from build123d import *

# Parameters (mm, degrees)
SKETCH1_W           = 48
SKETCH1_H           = 59
BOSS_EXTRUDE1_DEPTH = 2
BOSS_EXTRUDE2_DEPTH = 59
SKETCH3_W           = 14
SKETCH3_H           = 55.8
CUT_EXTRUDE1_DEPTH  = 13


with BuildPart() as part:
    # Sketch1 → Boss-Extrude1 (new body)
    with BuildSketch(Plane.XY):
        Rectangle(SKETCH1_W, SKETCH1_H)
    extrude(amount=BOSS_EXTRUDE1_DEPTH)

    # Sketch2 → Boss-Extrude2 (add)
    with BuildSketch(Plane.XZ.offset(29.5)):
        with BuildLine():
            Line((-16, 15), (16, 15))
            ThreePointArc((16, 15), (21.656854249, 12.656854249), (24, 7))
            Line((24, 7), (24, 2))
            Line((24, 2), (-24, 2))
            Line((-24, 2), (-24, 7))
            ThreePointArc((-24, 7), (-21.656854249, 12.656854249), (-16, 15))
        make_face()
    extrude(amount=-BOSS_EXTRUDE2_DEPTH)

    # Sketch3 → Cut-Extrude1 (cut)
    with BuildSketch(Plane.XY.offset(15)):
        Rectangle(SKETCH3_W, SKETCH3_H)
        with Locations((15.4, 0)):
            Rectangle(SKETCH3_W, SKETCH3_H)
        with Locations((-15.4, 0)):
            Rectangle(SKETCH3_W, SKETCH3_H)
    extrude(amount=-CUT_EXTRUDE1_DEPTH, mode=Mode.SUBTRACT)


solid = part.part
Verification items for the finished model (mm, model axes). A direction names the side the tool comes from. Round coordinates to 2 decimals unless told otherwise and drop trailing zeros. Loops run counter-clockwise (first coordinate to the right, second up) from the corner with the lowest first, then second, coordinate; pieces in that order, holes last. Notation, with made-up numbers: M -21.5,36 L 4.5,36 A20 cw 4.5,52 Z; hole C 53.25,8 d4. An arc over 180 degrees is marked long. Write each question's results on one line, items separated by ' | '.
1) Section check A-A on z = 3. Record the boundary of the cut face in (x, y), then the cut area to 3 significant figures.
Checks:
outline: M -24,-29.5 L 24,-29.5 L 24,29.5 L -24,29.5 Z; hole M -22.4,-27.9 L -8.4,-27.9 L -8.4,27.9 L -22.4,27.9 Z; hole M -7,-27.9 L 7,-27.9 L 7,27.9 L -7,27.9 Z; hole M 8.4,-27.9 L 22.4,-27.9 L 22.4,27.9 L 8.4,27.9 Z | area: 488 mm2
2) Mould release check, pull along Y, two halves, no side actions. Record for faces 3 (the flat face through (-24, 0, 3)), 4 (the flat face through (0, 29.5, 8)), 5 (the flat face through (15, 27.9, 9)): released by +Y, released by -Y, zero draft, split by the parting line, or undercut.
Checks:
face 3: zero draft | face 4: released by +Y | face 5: undercut
3) Access from +Z, -Z, +X, -X, +Y, -Y to the whole of each face (thin tool, end or side, straight path). Record for faces 1 (the flat face through (7, 0, 9)), 2 (the cylindrical face through (23.213, -0.413, 10.46)).
Checks:
face 1: +Z | face 2: +Z, +X, +Y, -Y
4) Gauge pin test, flat ends, axial feed: P1, Ø1, axis at x = 3.5, y = -8.5, coming from the -Z side; P2, Ø11, axis at x = 16.5, y = 2, coming from the +Z side. Record the tip position at first contact, or that the pin passes through.
Checks:
P1: stops at z = 0 | P2: stops at z = 2
5) Section check D-D on z = 12.75. Record the boundary of the cut face in (x, y).
Checks:
outline: M -21.56,-29.5 L 21.56,-29.5 L 21.56,-27.9 L 8.4,-27.9 L 8.4,27.9 L 21.56,27.9 L 21.56,29.5 L -21.56,29.5 L -21.56,27.9 L -8.4,27.9 L -8.4,-27.9 L -21.56,-27.9 Z; hole M -7,-27.9 L 7,-27.9 L 7,27.9 L -7,27.9 Z
6) Section check C-C on y = -14. Record the boundary of the cut face in (x, z), then the cut area to 3 significant figures.
Checks:
outline: M -24,0 L 24,0 L 24,7 A8 ccw 22.4,11.8 L 22.4,2 L 8.4,2 L 8.4,15 L 7,15 L 7,2 L -7,2 L -7,15 L -8.4,15 L -8.4,2 L -22.4,2 L -22.4,11.8 A8 ccw -24,7 Z | area: 159 mm2
7) Scan lines: L1, parallel to X at y = 20, z = 2.5; L2, parallel to Y at x = -20.5, z = 13.5; L3, parallel to X at y = 6, z = 13.5. Record each from-to range of solid material in increasing order. Write a range as from..to.
Checks:
L1: x = -24..-22.4, -8.4..-7, 7..8.4, 22.4..24 | L2: y = -29.5..-27.9, 27.9..29.5 | L3: x = -8.4..-7, 7..8.4
8) Section check B-B on x = 12. Record the boundary of the cut face in (y, z), then the cut area to 3 significant figures.
Checks:
outline: M -29.5,0 L 29.5,0 L 29.5,15 L 27.9,15 L 27.9,2 L -27.9,2 L -27.9,15 L -29.5,15 Z | area: 160 mm2
